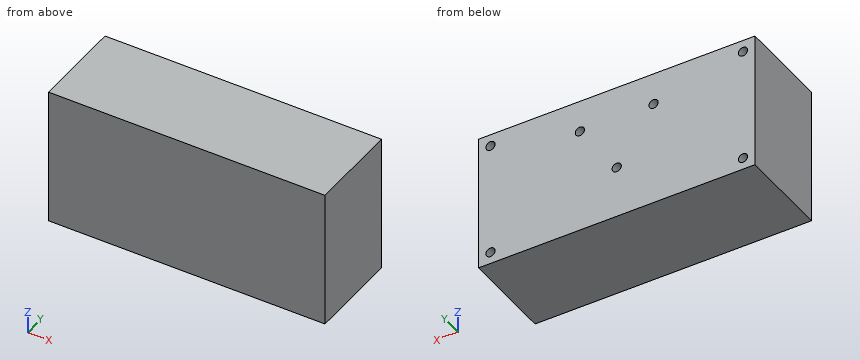
Autodesk Inventor part; units mm, degrees
ref_plane "YZ Plane" through (0, 0, 0) normal (1, 0, 0) x (0, 1, 0)
ref_plane "XZ Plane" through (0, 0, 0) normal (0, 1, 0) x (-1, 0, 0)
ref_plane "XY Plane" through (0, 0, 0) normal (0, 0, 1) x (1, 0, 0)
sketch "Sketch1" plane through (0, 0, 0) normal (0, 1, 0) x (-1, 0, 0)
  line L0 (0, -37.5) -> (-75, -37.5)
  line L1 (-75, -37.5) -> (-75, 0)
  line L2 (-75, 0) -> (0, 0)
  line L3 (0, 0) -> (0, -37.5)
  line L4 (-3.25, -34.25) -> (-71.75, -34.25) construction
  line L5 (-71.75, -34.25) -> (-71.75, -3.25) construction
  line L6 (-71.75, -3.25) -> (-3.25, -3.25) construction
  line L7 (-3.25, -3.25) -> (-3.25, -34.25) construction
  circle A0 centre (-3.25, -34.25) radius 1.25
  circle A1 centre (-37.5, -23.25) radius 1.25
  circle A2 centre (-3.25, -3.25) radius 1.25
  circle A3 centre (-71.75, -3.25) radius 1.25
  circle A4 centre (-71.75, -34.25) radius 1.25
  circle A5 centre (-47.5, -8.75) radius 1.25
  circle A6 centre (-27.5, -8.75) radius 1.25
  line L8 (-27.5, -8.75) -> (-47.5, -8.75) construction
  point P0 (-37.5, -34.25)
  point P1 (-37.5, -37.5)
  point P2 (-3.25, -18.75)
  point P3 (0, -18.75)
  point P4 (-37.5, -8.75)
  point P5 (-37.5, -3.25)
  dimension "d0" = 37.5
  dimension "d1" = 75
  dimension "d2" = 31
  dimension "d3" = 68.5
  dimension "d4" = 2.5
  dimension "d6" = 2.5
  dimension "d7" = 2.5
  dimension "d8" = 2.5
  dimension "d9" = 2.5
  dimension "d10" = 34.25
  dimension "d11" = 11
  dimension "d16" = 2.5
  dimension "d17" = 2.5
  dimension "d18" = 20
  dimension "d19" = 10
extrude "Extrusion1" add sketch "Sketch1" against normal blind 25 contours L0 L1 L2 L3 | A0 | A1 | A2 | A3 | A4 | A5 | A6
extrude "Extrusion2" cut sketch "Sketch1" against normal blind 8 contours A0 | A1 | A2 | A3 | A4 | A5 | A6
properties part number "heatsink-dual-CNC_3DPrint"
Verification items for the finished model (mm, model axes). Coordinates: 2 decimals unless noted, no trailing zeros. Write each loop counter-clockwise with the first axis right and the second up, starting at its lowest first coordinate (ties: lowest second). Pieces come first, ordered by that corner, then holes. Notation, with made-up numbers: (84.25, -20) -> (104.25, -20) arc R34 cw to (104.25, 15) -> close; hole circle Ø10 at (62, 85.5). An arc over 180 degrees is marked (long way). One line per item, written item: value. Start each with the question number.
Q1. Cross-section at C-C on x = 47.5. Enter the section's corners in (y, z), and give its area (4 significant figures).
Q2. Cross-section at B-B on x = 3.25. Enter the section's corners in (y, z), and give its area (4 significant figures).
Q3. Go/stop test with a flat-tipped pin: P1, Ø0.8, axis at x = 3, z = -3.5, coming from the +Y side. Record where the tip stops, or that it passes through.
Q4. Cross-section at A-A on z = -8.75. Enter the section's corners in (x, y).
Q5. Cross-section at D-D on x = 28. Enter the section's corners in (y, z), and give its area (3 significant figures).
Q6. Thickness scan on L1, parallel to Z at x = 3.25, y = -6.25; L2, parallel to Z at x = 71, y = -1.75; L3, parallel to X at y = -7.5, z = -35. Record the ranges inside material, lowest first. Write a range as from..to.
Checked values:
1. outline: (-25, -37.5) -> (0, -37.5) -> (0, -10) -> (-8, -10) -> (-8, -7.5) -> (0, -7.5) -> (0, 0) -> (-25, 0) -> close
1. area: 917.5 mm²
2. outline: (-25, -37.5) -> (0, -37.5) -> (0, -35.5) -> (-8, -35.5) -> (-8, -33) -> (0, -33) -> (0, -4.5) -> (-8, -4.5) -> (-8, -2) -> (0, -2) -> (0, 0) -> (-25, 0) -> close
2. area: 897.5 mm²
3. P1: stops at y = -8
4. outline: (0, -25) -> (75, -25) -> (75, 0) -> (48.75, 0) -> (48.75, -8) -> (46.25, -8) -> (46.25, 0) -> (28.75, 0) -> (28.75, -8) -> (26.25, -8) -> (26.25, 0) -> (0, 0) -> close
5. outline: (-25, -37.5) -> (0, -37.5) -> (0, -9.9) -> (-8, -9.9) -> (-8, -7.6) -> (0, -7.6) -> (0, 0) -> (-25, 0) -> close
5. area: 919 mm²
6. L1: z = -37.5..-35.5, -33..-4.5, -2..0
6. L2: z = -37.5..-35.25, -33.25..-4.25, -2.25..0
6. L3: x = 0..2.25, 4.25..70.75, 72.75..75
